from build123d import *

# Parameters (mm, degrees)
ESQUISSE1_R             = 2.5
BOSS_EXTRU_1_DEPTH      = 3
ESQUISSE2_W             = 20
ESQUISSE2_H             = 10
ENL_V_MAT_EXTRU_1_DEPTH = 174.720827721


with BuildPart() as part:
    # Esquisse1 → Boss.-Extru.1 (new body)
    with BuildSketch(Plane(origin=(0, 0, 0), x_dir=(1, 0, 0), z_dir=(0, 1, 0))):
        Polygon((-170.028456395, 18.77), (-170.028456395, -23), (-170.028456395, -35.5), (110.271543605, -35.5), (110.271543605, -10.5), (65.057787015, -10.5), (65.057787015, 28.77), (-170.028456395, 28.77), align=None)
        with Locations(Location((100.471543605, -23, 0), (0, 0, 270))):
            Circle(ESQUISSE1_R, mode=Mode.SUBTRACT)
        with Locations(Location((-160.228456395, -19.4325, 0), (0, 0, 270))):
            Circle(ESQUISSE1_R, mode=Mode.SUBTRACT)
        with Locations(Location((-160.228456395, 12.7025, 0), (0, 0, 270))):
            Circle(ESQUISSE1_R, mode=Mode.SUBTRACT)
        with Locations(Location((45.007787015, 10.635, 0), (0, 0, 270))):
            Circle(ESQUISSE1_R, mode=Mode.SUBTRACT)
    extrude(amount=BOSS_EXTRU_1_DEPTH)

    # Esquisse2 → Enlèv. mat.-Extru.1 (cut, through all)
    with BuildSketch(Plane(origin=(0, 3, 0), x_dir=(1, 0, 0), z_dir=(0, 1, 0))):
        with BuildLine():
            Line((-118.756895542, 11.635), (-118.756895542, -18.365))
            ThreePointArc((-118.756895542, -18.365), (-111.256895542, -25.865), (-103.756895542, -18.365))
            Line((-103.756895542, -18.365), (-103.756895542, 11.635))
            ThreePointArc((-103.756895542, 11.635), (-111.256895542, 19.135), (-118.756895542, 11.635))
        make_face()
        with BuildLine():
            Line((-59.98533469, 11.635), (-59.98533469, -18.365))
            ThreePointArc((-59.98533469, -18.365), (-52.48533469, -25.865), (-44.98533469, -18.365))
            Line((-44.98533469, -18.365), (-44.98533469, 11.635))
            ThreePointArc((-44.98533469, 11.635), (-52.48533469, 19.135), (-59.98533469, 11.635))
        make_face()
        with BuildLine():
            Line((-1.213773837, 11.635), (-1.213773837, -18.365))
            ThreePointArc((-1.213773837, -18.365), (6.286226163, -25.865), (13.786226163, -18.365))
            Line((13.786226163, -18.365), (13.786226163, 11.635))
            ThreePointArc((13.786226163, 11.635), (6.286226163, 19.135), (-1.213773837, 11.635))
        make_face()
        with Locations((75.271543605, -23)):
            Rectangle(ESQUISSE2_W, ESQUISSE2_H)
    extrude(amount=-ENL_V_MAT_EXTRU_1_DEPTH, mode=Mode.SUBTRACT)


solid = part.part
Geometry check sheet. Reference: the model listing, model coordinates, mm. A direction names the side the tool comes from. Coordinates: 2 decimals unless noted, no trailing zeros. One line per question, with ' | ' between items.
1. Cross-section at A-A on y = 1.3. State how many separate pieces and enclosed holes the cut face has, and give its area (3 significant figures).
Answers:
separate pieces: 1 | enclosed holes: 8 | area: 14,100 mm²
2. Set-up check for faces 1 (the cylindrical face through (6.121, 1.521, 25.863)), 2 (the flat face through (-32, 3, 3)): record each of +Z, -Z, +X, -X, +Y, -Y from which the full face is reachable in a straight line by a thin tool's end or side.
Answers:
face 1: +Y, -Y | face 2: +Z, -Z, +X, -X, +Y
3. Thickness scan on probe 1 along X at (y, z) = (0.25, 14); probe 2 along X at (y, z) = (1.6, -0.5); probe 3 along Z at (x, y) = (81, 2.6). Record the ranges inside material, lowest first. Write a range as from..to.
Answers:
probe 1: x = -170.03..-118.76, -103.76..-59.99, -44.99..-1.21, 13.79..110.27 | probe 2: x = -170.03..-118.76, -103.76..-59.99, -44.99..-1.21, 13.79..65.06 | probe 3: z = 10.5..18, 28..35.5
4. Draft check along X on faces 3 (the flat face through (-32, 0, 3)), 4 (the cylindrical face through (-162.446, 1.479, 20.586)). Enter one of: +X half, -X half, draft (parallel to the pull), parting line (faces both ways), or undercut.
Answers:
face 3: draft | face 4: undercut
5. Depth check by flat-ended pin: pin 1 Ø1.5 at (y, z) = (2, -2) entering from +X; pin 2 Ø1.5 at (x, y) = (95.5, 2) entering from -Z. Enter the tip coordinate at first touch or a pass-through.
Answers:
pin 1: stops at x = 65.06 | pin 2: stops at z = 10.5
